The model under review builds one solid part; all positions refer to its coordinate system, in mm. Coordinates: 2 decimals unless noted, no trailing zeros. Loops run counter-clockwise (first coordinate to the right, second up) from the corner with the lowest first, then second, coordinate; pieces in that order, holes last. Notation, with made-up numbers: (-39.75, 66.5) - (-16.75, 66.5) arc R17 cw to (-16.75, 84.5) - close; hole circle Ø5 at (-24, -24.75). An arc over 180 degrees is marked (long way). Use a Markdown table: item, result. Add a question column.
1) The part is to be moulded in two halves that separate along Y. For faces 1 (the cylindrical face through (23.846, -7.509, -0.07)), 2 (the flat face through (-59, 4, 5)), say which applies: pulls with the +Y half, pulls with the -Y half, needs draft (parallel to the pull), parting line crosses it, or undercut.
2) To check wall thickness, follow L1, parallel to Y at x = 0, z = 1; L2, parallel to Y at x = -4, z = 3; L3, parallel to X at y = 3, z = 0. State the ranges of each line that lie inside material, in increasing order. Write a range as [from, to].
3) Add section A-A, the plane x = 0. Give the boundary of the cut face in (y, z), and give its area (3 significant figures).
Autodesk Fusion 360 part; units mm, degrees
sketch "Sketch1" plane through (0, 0, 0) normal (0, 0, 1) x (1, 0, 0)
  circle A0 centre (0, 0) radius 25
  line L0 (-250, 250) -> (250, 250)
  line L1 (250, 250) -> (250, -250)
  line L2 (250, -250) -> (-250, -250)
  line L3 (-250, -250) -> (-250, 250)
  line L4 (-250, 0) -> (250, 0) construction
  line L5 (0, -250) -> (0, 250) construction
  dimension "Total_Width" = 500
  dimension "Hole_Radius" = 25
extrude "Extrude1" add sketch "Sketch1" along normal mid plane 10
From the geometry:
| question | item | result |
|---|---|---|
| 1 | face 1 | undercut |
| 1 | face 2 | needs draft |
| 2 | L1 | y = [-250, -25], [25, 250] |
| 2 | L2 | y = [-250, -24.68], [24.68, 250] |
| 2 | L3 | x = [-250, -24.82], [24.82, 250] |
| 3 | outline | (-250, -5) - (-25, -5) - (-25, 5) - (-250, 5) - close; (25, -5) - (250, -5) - (250, 5) - (25, 5) - close |
| 3 | area | 4,500 mm^2 |
